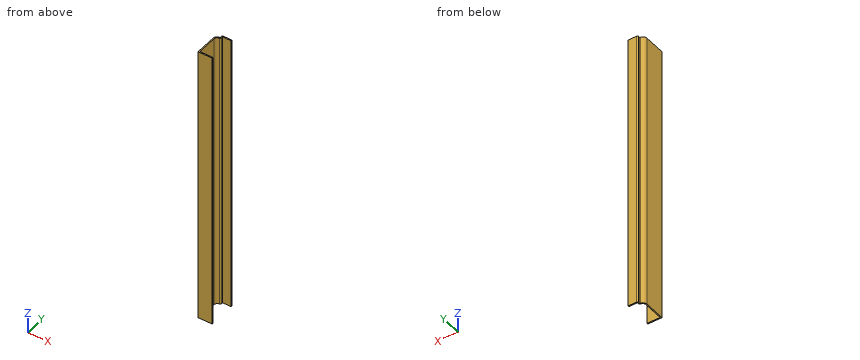
from build123d import *

# Parameters (mm, degrees)
EXTRUDE_THIN1_DEPTH = 317.5
FILLET1_R           = 1.27


with BuildPart() as part:
    # Sketch1 → Extrude-Thin1 (new body)
    with BuildSketch(Plane.XY):
        with BuildLine():
            Line((0, 0), (-15.875, 0))
            Line((-15.875, 0), (-15.875, 23.8125))
            ThreePointArc((-15.875, 23.8125), (-14.480096045, 27.180096045), (-11.1125, 28.575))
            Line((-11.1125, 28.575), (-11.1125, 31.75))
            Line((-11.1125, 31.75), (0, 31.75))
            Line((0, 31.75), (0, 30.48))
            Line((0, 30.48), (-9.8425, 30.48))
            Line((-9.8425, 30.48), (-9.8425, 27.065906868))
            ThreePointArc((-9.8425, 27.065906868), (-13.082535691, 26.696336962), (-14.605, 23.8125))
            Line((-14.605, 23.8125), (-14.605, 1.27))
            Line((-14.605, 1.27), (0, 1.27))
            Line((0, 1.27), (0, 0))
        make_face()
    extrude(amount=-EXTRUDE_THIN1_DEPTH)

    # Fillet1
    fillet1_edges = [part.edges().sort_by_distance(p)[0] for p in [
        (-9.8425, 27.065906868, -158.75),
        (-11.1125, 31.75, -158.75),
    ]]
    fillet(fillet1_edges, radius=FILLET1_R)


solid = part.part
Check sheet for the modelled part. Datum: model origin and axes. Units: mm. Round coordinates to 2 decimals unless told otherwise and drop trailing zeros. Write each loop counter-clockwise with the first axis right and the second up, starting at its lowest first coordinate (ties: lowest second). Pieces come first, ordered by that corner, then holes. Notation, with made-up numbers: (10.25, -23) - (46.25, -23) arc R35 cw to (46.25, 16) - close; hole circle Ø3 at (10, -10). An arc over 180 degrees is marked (long way). Return JSON: item names as keys, results as strings.
Q1. Scan lines: L1, parallel to Y at x = -4, z = -184.5; L2, parallel to X at y = 14, z = -156 (3 decimals); L3, parallel to Y at x = -11.5, z = -234. Record each from-to range of solid material in increasing order. Write a range as from..to.
Returned:
{"L1": "y = 0..1.27, 30.48..31.75", "L2": "x = -15.875..-14.605", "L3": "y = 0..1.27, 27.28..28.56"}
Q2. Cross-section at A-A (x = -3.5). Record the boundary of the cut face in (y, z).
Returned:
{"outline": "(0, -317.5) - (1.27, -317.5) - (1.27, 0) - (0, 0) - close; (30.48, -317.5) - (31.75, -317.5) - (31.75, 0) - (30.48, 0) - close"}
Q3. Cross-section at C-C (y = 20). Record the boundary of the cut face in (x, z) (3 decimals).
Returned:
{"outline": "(-15.875, -317.5) - (-14.605, -317.5) - (-14.605, 0) - (-15.875, 0) - close"}
Q4. Depth check by flat-ended pin: P1, Ø7, axis at y = 15.5, z = -188, coming from the +X side (3 decimals); P2, Ø2, axis at x = -7.5, z = -124.5, coming from the -Y side; P3, Ø1.5, axis at y = 30, z = -237.5, coming from the -X side. Enter the tip coordinate at first touch or a pass-through.
Returned:
{"P1": "stops at x = -14.605", "P2": "stops at y = 0", "P3": "stops at x = -11.11"}
